Source: CAD feature listing. Evaluate the final solid. Frame: model axes, mm. Coordinates: 2 decimals unless noted, no trailing zeros. Order: outer loops, then holes, each group sorted by start corner. A loop starts at its lowest first (then second) coordinate and runs counter-clockwise, first axis right, second up.
Item 1: Ray query, line 1 (X direction, y = 27.5, z = 1.2). Return the intervals inside material, ascending.
Item 2: Contact query for flat-ended pins moving along their axis: P1, Ø1.5, axis at y = 19, z = 0.5, coming from the -X side; P2, Ø1.5, axis at x = 253, z = -0.5, coming from the -Y side; P3, Ø2, axis at y = 41, z = 1, coming from the +X side. Output: stop coordinate, or through.
Item 3: Section B-B on y = -23.5. Return the cut outline in (x, z).
from build123d import *

# Parameters (mm, degrees)
BOSS_EXTRUDE1_DEPTH = 2.5
FILLET1_R           = 3.175


with BuildPart() as part:
    # Sketch1 → Boss-Extrude1 (new, symmetric)
    with BuildSketch(Plane.XY):
        Polygon((-260.35, 68.2625), (260.35, 68.2625), (260.35, 42.8625), (239.7125, 42.8625), (239.7125, -42.8625), (-239.7125, -42.8625), (-239.7125, 42.8625), (-260.35, 42.8625), align=None)
    extrude(amount=BOSS_EXTRUDE1_DEPTH, both=True)

    # Fillet1
    fillet1_edges = [part.edges().sort_by_distance(p)[0] for p in [
        (-260.35, 68.2625, 0),
        (260.35, 68.2625, 0),
        (260.35, 42.8625, 0),
        (-260.35, 42.8625, 0),
    ]]
    fillet(fillet1_edges, radius=FILLET1_R)


solid = part.part
Answer list:
1. line 1: x = -239.71 to 239.71
2. P1: stops at x = -239.71
2. P2: stops at y = 42.86
2. P3: stops at x = 239.71
3. outline: (-239.71, -2.5) - (239.71, -2.5) - (239.71, 2.5) - (-239.71, 2.5) - close
